Part print with two shaded views. Sizes in mm from the minimum x, y, z corner. A direction names the side the tool comes from. Round coordinates to 2 decimals unless told otherwise and drop trailing zeros. Loops run counter-clockwise (first coordinate to the right, second up) from the corner with the lowest first, then second, coordinate; pieces in that order, holes last. Notation, with made-up numbers: (42, 28) -> (79, 28) arc R25 ccw to (79, 45) -> close; hole circle Ø10 at (77, 16.5). An arc over 180 degrees is marked (long way). Answer as a JSON object with one key per item and string values. Group by question number.
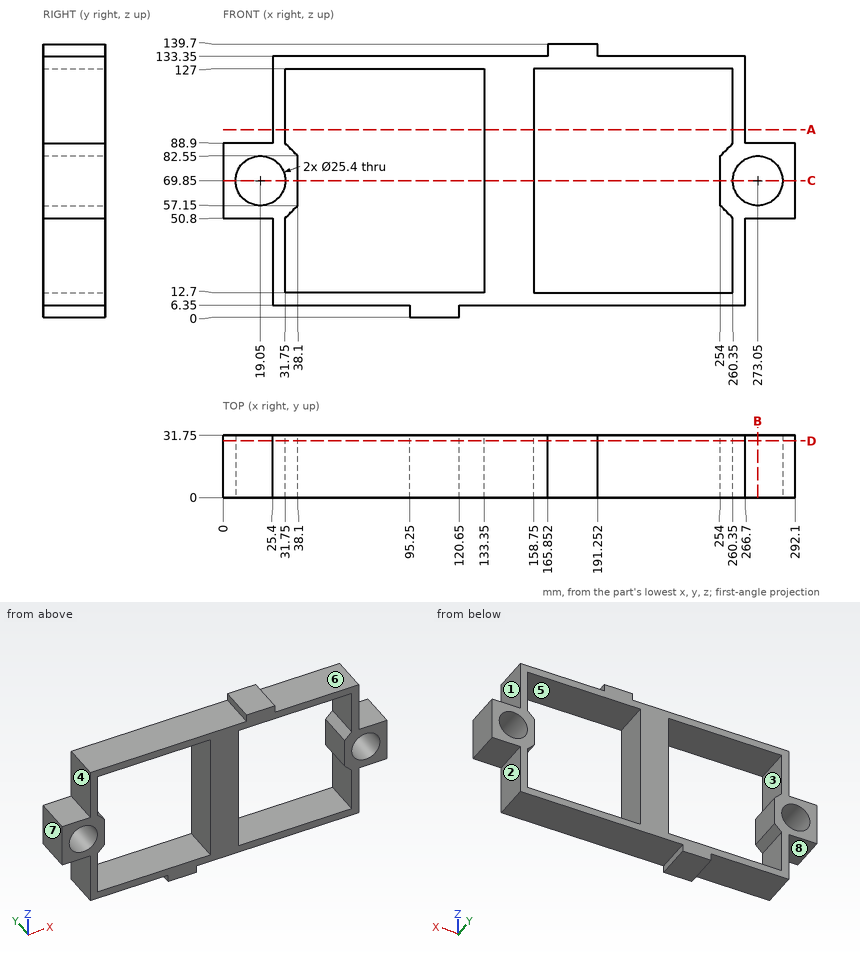
Item 1: Two-plate mould, pull along Z, no slides. Class the marked faces 5, 6, 7 and 8: pulls with the +Z half, pulls with the -Z half, needs draft (parallel to the pull), parting line crosses it, or undercut.
Item 2: Band-saw the part on B-B, the plane x = 273.05. List the corners of the cut face in (y, z), plus the area to 3 significant figures.
Item 3: Band-saw the part on D-D, the plane y = 29. Count the separate pieces of the cut face and the enclosed holes in it, plus the area to 3 significant figures.
Item 4: Band-saw the part on A-A, the plane z = 96. List the corners of the cut face in (x, y).
Item 5: Band-saw the part on C-C, the plane z = 69.85. List the corners of the cut face in (x, y).
Item 6: Drill centre lines: line 1 (X direction, y = 15, z = 105); line 2 (X direction, y = 23, z = 69); line 3 (Z direction, x = 252, y = 19.5). Where is each one in solid material? Low to high.
Item 7: Which spindle directions (+Z, -Z, +X, -X, +Y, -Y) get a long thin tool onto all of the face, cutting with end or side? Do the marked faces 1, 2, 3 and 4. Say none if no direction does.
Item 8: Drop flat-ended pins along their axis: pin 1 Ø16 at (x, y) = (185.5, 12) entering from -Z; pin 2 Ø16 at (x, y) = (224, 12.5) entering from +Z; pin 3 Ø20.5 at (x, z) = (273.05, 69.85) entering from -Y; pin 4 Ø10 at (y, z) = (14.5, 36) entering from -X. Give the stop position or say it passes through.
Entries:
{
 "1": {"face 5": "undercut", "face 6": "pulls with the +Z half", "face 7": "needs draft", "face 8": "pulls with the -Z half"},
 "2": {"outline": "(0, 50.8) -> (31.75, 50.8) -> (31.75, 57.15) -> (0, 57.15) -> close; (0, 82.55) -> (31.75, 82.55) -> (31.75, 88.9) -> (0, 88.9) -> close", "area": "403 mm²"},
 "3": {"separate pieces": "1", "enclosed holes": "4", "area": "9,070 mm²"},
 "4": {"outline": "(25.4, 0) -> (31.75, 0) -> (31.75, 31.75) -> (25.4, 31.75) -> close; (133.35, 0) -> (158.75, 0) -> (158.75, 31.75) -> (133.35, 31.75) -> close; (260.35, 0) -> (266.7, 0) -> (266.7, 31.75) -> (260.35, 31.75) -> close"},
 "5": {"outline": "(0, 0) -> (6.35, 0) -> (6.35, 31.75) -> (0, 31.75) -> close; (31.75, 0) -> (38.1, 0) -> (38.1, 31.75) -> (31.75, 31.75) -> close; (133.35, 0) -> (158.75, 0) -> (158.75, 31.75) -> (133.35, 31.75) -> close; (254, 0) -> (260.35, 0) -> (260.35, 31.75) -> (254, 31.75) -> close; (285.75, 0) -> (292.1, 0) -> (292.1, 31.75) -> (285.75, 31.75) -> close"},
 "6": {"line 1": "25.4 to 31.75, 133.35 to 158.75, 260.35 to 266.7", "line 2": "0 to 6.38, 31.72 to 38.1, 133.35 to 158.75, 254 to 260.38, 285.72 to 292.1", "line 3": "6.35 to 12.7, 127 to 133.35"},
 "7": {"face 1": "+Z, +X, +Y, -Y", "face 2": "-Z, +X, +Y, -Y", "face 3": "+Y, -Y", "face 4": "+Z, -X, +Y, -Y"},
 "8": {"pin 1": "z = 6.35", "pin 2": "z = 133.35", "pin 3": "through", "pin 4": "x = 25.4"}
}
